Study the drawing (mm; zero at the part's minimum x, y, z) and answer. A direction names the side the tool comes from. Round coordinates to 2 decimals unless told otherwise and drop trailing zeros. Write each loop counter-clockwise with the first axis right and the second up, starting at its lowest first coordinate (ties: lowest second). Pieces come first, ordered by that corner, then holes.
(1) A cutting plane is placed at C-C, the plane z = 3.75. Give the vertices of the cut face in (x, y), and give its area (3 significant figures).
(2) Each of these flat-tipped pins is pushed along its axis until it touches: pin 1 Ø6 at (y, z) = (7.5, 3) entering from -X; pin 2 Ø1.7 at (x, y) = (12.5, 20.5) entering from -Z; pin 3 Ø1.4 at (x, y) = (12.5, 3) entering from +Z. Where does it stop, or does it pass through?
(3) For the marked faces 3, 4 and 5, determine the directions among +Z, -Z, +X, -X, +Y, -Y from which every point of the face is accessible in a straight line to the end or side of a thin tool.
(4) The mould has two halves that part along Y. Classify the marked faces 1 and 2: +Y half, -Y half, draft (parallel to the pull), parting line (faces both ways), or undercut.
(5) A cutting plane is placed at A-A, the plane x = 12.5. Give the vertices of the cut face in (y, z) (3 decimals).
(6) Find the intervals of material crossed by probe 1 along Y at (x, z) = (12.5, 1); probe 2 along Y at (x, z) = (12.5, 11.45) (3 decimals); probe 3 along X at (y, z) = (12.75, 10.5), in increasing order.
(7) A cutting plane is placed at D-D, the plane y = 3.75. Give the vertices of the cut face in (x, z), and give its area (3 significant figures).
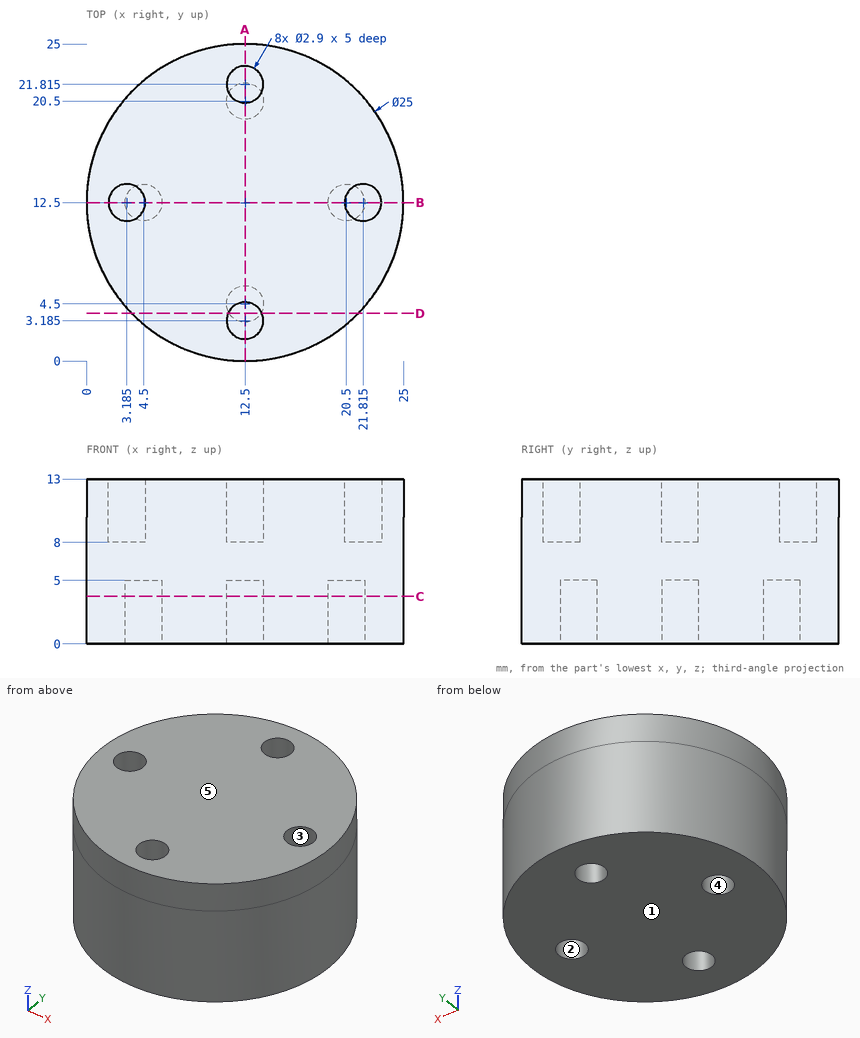
Solutions:
1. outline: circle Ø25 at (12.5, 12.5); hole circle Ø2.9 at (4.5, 12.5); hole circle Ø2.9 at (12.5, 4.5); hole circle Ø2.9 at (12.5, 20.5); hole circle Ø2.9 at (20.5, 12.5)
1. area: 464 mm2
2. pin 1: stops at x = 0.16
2. pin 2: stops at z = 5
2. pin 3: stops at z = 8
3. face 3: +Z
3. face 4: -Z
3. face 5: +Z, +X, -X, +Y, -Y
4. face 1: draft
4. face 2: undercut
5. outline: (0, 0) - (3.05, 0) - (3.05, 5) - (5.95, 5) - (5.95, 0) - (19.05, 0) - (19.05, 5) - (21.95, 5) - (21.95, 0) - (25, 0) - (25, 13) - (23.265, 13) - (23.265, 8) - (20.365, 8) - (20.365, 13) - (4.635, 13) - (4.635, 8) - (1.735, 8) - (1.735, 13) - (0, 13) - close
6. probe 1: y = 0 to 3.05, 5.95 to 19.05, 21.95 to 25
6. probe 2: y = 0 to 1.735, 4.635 to 20.365, 23.265 to 25
6. probe 3: x = 0 to 1.76, 4.61 to 20.39, 23.24 to 25
7. outline: (3.57, 0) - (11.26, 0) - (11.26, 5) - (13.74, 5) - (13.74, 0) - (21.43, 0) - (21.43, 13) - (13.84, 13) - (13.84, 8) - (11.16, 8) - (11.16, 13) - (3.57, 13) - close
7. area: 206 mm2
